Check sheet for the modelled part. Datum: model origin and axes. Units: mm. A direction names the side the tool comes from. Coordinates: 2 decimals unless noted, no trailing zeros. Loops run counter-clockwise (first coordinate to the right, second up) from the corner with the lowest first, then second, coordinate; pieces in that order, holes last. Notation, with made-up numbers: (8.5, 8.5) - (18.5, 8.5) arc R35 ccw to (18.5, 40.5) - close; hole circle Ø4 at (51.5, 68.25). An arc over 180 degrees is marked (long way). Write each question's results on one line, items separated by ' | '. Start each with the question number.
1. Cross-section at A-A (x = 5). Record the cut outline in (y, z), and give its area (4 significant figures).
2. Cross-section at C-C (y = -4.25). Record the cut outline in (x, z).
3. Cross-section at B-B (z = 33.25). Record the cut outline in (x, y), and give its area (3 significant figures).
4. Tool access check on faces 4 (the face through (0, -15, 5)), 5 (the face through (5, 4, -19.25)), 6 (the face through (5, 2, -22)). Record the directions out of +Z, -Z, +X, -X, +Y, -Y that give a thin tool (end or side, any length) a straight path to the whole face; none if there is none.
5. Gauge pin test, flat ends, axial feed: P1, Ø3, axis at x = -3, z = -21.5, coming from the -Y side; P2, Ø1, axis at y = -6.5, z = 0, coming from the +X side; P3, Ø6.5, axis at y = 1.5, z = 29, coming from the -X side; P4, Ø5, axis at x = 7, z = 21.5, coming from the -Y side. Record the tip position at first contact, or that the pin passes through.
6. Thickness scan on line 1 (Z direction, x = 5, y = 0); line 2 (Z direction, x = 8, y = -0.75); line 3 (Z direction, x = 5, y = 3.5). Record the ranges inside material, lowest first. Write a range as [from, to].
7. Cross-section at D-D (z = -6.5). Record the cut outline in (x, y), and give its area (3 significant figures).
8. Draft check along X on faces 1 (the face through (4.566, 0.944, 31.298)), 2 (the face through (5, 0, -25.25)), 3 (the face through (10, -2.3, 12.9)). Enter one of: released by +X, released by -X, zero draft, split by the parting line, or undercut.
Autodesk Inventor part; units mm, degrees
ref_plane "YZ Plane" through (0, 0, 0) normal (1, 0, 0) x (0, 1, 0)
ref_plane "XZ Plane" through (0, 0, 0) normal (0, 1, 0) x (-1, 0, 0)
ref_plane "XY Plane" through (0, 0, 0) normal (0, 0, 1) x (1, 0, 0)
sketch "Эскиз1" plane through (0, 0, 0) normal (1, 0, 0) x (0, 1, 0)
  line L0 (-2, 25.25) -> (2, 25.25)
  line L1 (2, 25.25) -> (2, -25.25)
  line L2 (2, -25.25) -> (-2, -25.25)
  line L3 (-2, -25.25) -> (-2, 25.25)
  line L4 (-2, 25.25) -> (2, -25.25) construction
  line L5 (2, 25.25) -> (-2, -25.25) construction
  line L6 (2, 25.25) -> (5, 25.25)
  line L7 (5, 25.25) -> (5, 19.25)
  line L8 (5, 19.25) -> (2, 19.25)
  line L9 (2, 19.25) -> (2, 25.25)
  line L10 (2, -25.25) -> (5, -25.25)
  line L11 (5, -25.25) -> (5, -19.25)
  line L12 (5, -19.25) -> (2, -19.25)
  line L13 (2, -19.25) -> (2, -25.25)
  line L14 (5, 25.25) -> (-5, 25.25)
  line L15 (-5, 25.25) -> (-5, 28.25)
  line L16 (-5, 28.25) -> (5, 28.25)
  line L17 (5, 28.25) -> (5, 25.25)
  line L18 (5, -25.25) -> (-5, -25.25)
  line L19 (-5, -25.25) -> (-5, -28.25)
  line L20 (-5, -28.25) -> (5, -28.25)
  line L21 (5, -28.25) -> (5, -25.25)
  line L22 (-5, 28.25) -> (-2, 28.25)
  line L23 (-2, 28.25) -> (-2, -28.25)
  line L24 (-2, -28.25) -> (-5, -28.25)
  line L25 (-5, -28.25) -> (-5, 28.25)
  point P0 (0, 0)
  dimension "d0" = 4
  dimension "d1" = 50.5
  dimension "d2" = 3
  dimension "d3" = 6
  dimension "d4" = 3
  dimension "d5" = 6
  dimension "d6" = 10
  dimension "d7" = 10
  dimension "d8" = 3
  dimension "d9" = 3
extrude "Выдавливание1" add sketch "Эскиз1" along normal blind 10 contours L23 L16 L17 L6 L0 | L3 L18 L25 L14 | L14 L15 L16 L23 | L6 L7 L8 L1 | L23 L20 L19 L18 | L2 L10 L21 L20 L23 | L1 L12 L11 L10
sketch "Эскиз2" plane through (0, -5, -28.25) normal (0, -1, 0) x (1, 0, 0)
  line L0 (10, 47.5) -> (10, 56.5)
  line L1 (10, 56.5) -> (0, 56.5)
  line L2 (0, 56.5) -> (0, 66.5)
  line L3 (0, 66.5) -> (10, 66.5)
  line L4 (10, 66.5) -> (10, 56.5)
  circle A0 centre (5, 61.5) radius 2
  line L5 (0, 61.5) -> (3, 61.5)
  line L6 (7, 61.5) -> (10, 61.5)
  point P0 (0, 28.25)
  dimension "d14" = 10
  dimension "d15" = 10
  dimension "d29" = 4
  dimension "d30" = 5
  dimension "d31" = 5
extrude "Выдавливание2" add sketch "Эскиз2" against normal blind 10 contours L1 L2 L5 A0 L6 L4 | L6 A0 L5 L2 L3 L4
sketch "Эскиз3" plane through (0, -5, -28.25) normal (0, -1, 0) x (1, 0, 0)
  line L0 (0, 56.5) -> (10, 56.5)
  line L1 (0, 56.5) -> (-7, 56.5)
  line L2 (-7, 56.5) -> (-7, 10.5)
  line L3 (-7, 10.5) -> (0, 10.5)
  line L4 (0, 10.5) -> (0, 56.5)
  point P0 (0, 28.25)
  dimension "d21" = 7
extrude "Выдавливание3" add sketch "Эскиз3" along normal blind 20 and the other way blind 1
sketch "Эскиз4" plane through (0, -5, -28.25) normal (0, -1, 0) x (1, 0, 0)
  line L0 (10, 47.5) -> (10, 56.5)
  line L1 (10, 56.5) -> (0, 56.5)
  line L2 (0, 56.5) -> (0, 66.5)
  line L3 (0, 66.5) -> (10, 66.5)
  line L4 (10, 66.5) -> (10, 56.5)
  circle A0 centre (5, 61.5) radius 2
  line L5 (0, 61.5) -> (3, 61.5)
  line L6 (7, 61.5) -> (10, 61.5)
  point P0 (0, 28.25)
  point P1 (0, 28.25)
  dimension "d32" = 10
  dimension "d33" = 10
  dimension "d34" = 4
  dimension "d35" = 5
  dimension "d36" = 5
extrude "Выдавливание4" cut sketch "Эскиз4" against normal blind 2 contours L1 L2 L5 A0 L6 L4 | L6 A0 L5 L2 L3 L4
move faces "Перенос1" translate (0, 2, 0) faces at (-2.3333, -4, -2.4167) (0, -11.6667, -2.4167)
properties part number "000.702 - Активный прижим" material "Пластик АБС"
Established:
1) outline: (-5, -28.25) - (5, -28.25) - (5, -19.25) - (2, -19.25) - (2, -25.25) - (-2, -25.25) - (-2, 25.25) - (2, 25.25) - (2, 19.25) - (5, 19.25) - (5, 31.25) - (-3, 31.25) - (-3, 28.25) - (-5, 28.25) - close; (-3, 35.25) - (5, 35.25) - (5, 38.25) - (-3, 38.25) - close | area: 295.5 mm^2
2) outline: (-7, -17.75) - (0, -17.75) - (0, -28.25) - (10, -28.25) - (10, 28.25) - (-7, 28.25) - close
3) outline: (0, -3) - (3, -3) - (3, 5) - (0, 5) - close; (7, -3) - (10, -3) - (10, 5) - (7, 5) - close | area: 48.0 mm^2
4) face 4: +Z, -Z, +X, -Y | face 5: +X, -X, +Y | face 6: +X, -X
5) P1: through | P2: x = 0 | P3: x = 0 | P4: y = -5
6) line 1: [-28.25, -25.25], [25.25, 31.25], [35.25, 38.25] | line 2: [-28.25, -25.25], [25.25, 38.25] | line 3: [-28.25, -19.25], [19.25, 31.25], [35.25, 38.25]
7) outline: (-7, -25) - (0, -25) - (0, -5) - (10, -5) - (10, -2) - (-7, -2) - close | area: 191 mm^2
8) face 1: undercut | face 2: zero draft | face 3: released by +X
